from build123d import *

# Parameters (mm, degrees)
SKETCH1_R           = 3.175
BOSS_EXTRUDE1_DEPTH = 66.04
BOSS_EXTRUDE2_START = -2.54
BOSS_EXTRUDE2_DEPTH = 2.54
SKETCH3_R           = 6.35
SKETCH3_R_2         = 3.175
BOSS_EXTRUDE3_DEPTH = 6.35


with BuildPart() as part:
    # Sketch1 → Boss-Extrude1 (new body)
    with BuildSketch(Plane(origin=(0, 0, 0), x_dir=(1, 0, 0), z_dir=(0, 1, 0))):
        with Locations(Location((0, 0, 0), (0, 0, 270))):
            Circle(SKETCH1_R)
    extrude(amount=BOSS_EXTRUDE1_DEPTH)

    # Sketch2 → Boss-Extrude2 (add)
    with BuildSketch(Plane(origin=(0, 66.04, 0), x_dir=(1, 0, 0), z_dir=(0, 1, 0)).offset(BOSS_EXTRUDE2_START)):
        with BuildLine():
            Line((1.27, 4.259709497), (1.27, 2.909935566))
            ThreePointArc((1.27, 2.909935566), (0, 3.175), (-1.27, 2.909935566))
            Line((-1.27, 2.909935566), (-1.27, 4.259709497))
            ThreePointArc((-1.27, 4.259709497), (0, 4.445), (1.27, 4.259709497))
        make_face()
    extrude(amount=BOSS_EXTRUDE2_DEPTH)

    # Sketch3 → Boss-Extrude3 (add)
    with BuildSketch(Plane.XZ):
        with Locations(Location((0, 0, 0), (0, 0, 270))):
            Circle(SKETCH3_R)
        with Locations(Location((0, 0, 0), (0, 0, 270))):
            Circle(SKETCH3_R_2, mode=Mode.SUBTRACT)
    extrude(amount=-BOSS_EXTRUDE3_DEPTH)


solid = part.part
Part model, mm, in its own coordinate system. A direction names the side the tool comes from. Give positions to 0.01 mm unless a question says otherwise; leave off trailing zeros. Order: outer loops, then holes, each group sorted by start corner. A loop starts at its lowest first (then second) coordinate and runs counter-clockwise, first axis right, second up. Notation, with made-up numbers: (-21, -0.5) -> (21, -0.5) arc R13 cw to (21, 24.5) -> close; hole circle Ø3 at (34, 50). An arc over 180 degrees is marked (long way). Use one line per item in the form item = value.
(1) Saw through at A-A (x = 0). Write the cut outline in (y, z) (3 decimals).
Solution:
outline = (0, -6.35) -> (6.35, -6.35) -> (6.35, -3.175) -> (63.5, -3.175) -> (63.5, -4.445) -> (66.04, -4.445) -> (66.04, 3.175) -> (6.35, 3.175) -> (6.35, 6.35) -> (0, 6.35) -> close
(2) Saw through at C-C (y = 16.5). Write the cut outline in (x, z) (3 decimals).
Solution:
outline = circle Ø6.35 at (0, 0)
(3) Tool access for faces 4 (the face through (1.27, 65, -4)), 5 (the face through (0, 0, 0)), 6 (the face through (-1.27, 65, -4)): list every direction of +Z, -Z, +X, -X, +Y, -Y with a clear straight run to the whole face (end or side of a thin tool).
Solution:
face_4 = -Z, +X, +Y
face_5 = +Z, -Z, +X, -X, -Y
face_6 = -Z, -X, +Y
(4) Pull direction Y, two halves, no side cores. Call faces 1 (the face through (-0.018, 64.752, -4.445)), 2 (the face through (0, 66.04, -1)), 3 (the face through (0, 63.5, -4)): +Y half, -Y half, draft (parallel to the pull), parting line (faces both ways), or undercut.
Solution:
face_1 = draft
face_2 = +Y half
face_3 = undercut
(5) Flat gauge pins, fed straight in: P1, Ø4, axis at y = 10, z = -4.5, coming from the +X side; P2, Ø1.5, axis at x = 2.5, y = 15, coming from the +Z side; P3, Ø1, axis at x = 1, y = 35.5, coming from the -Z side. Where does each tip first touch, or does it go through?
Solution:
P1 = 1.96
P2 = 2.65
P3 = -3.14
(6) Drill centre lines: line 1 (Y direction, x = -0.5, z = 4.25); line 2 (X direction, y = 25, z = -0.25); line 3 (X direction, y = 34, z = 0.75). Where is each one in solid material? Low to high. Write a range as from..to.
Solution:
line_1 = 0..6.35
line_2 = -3.17..3.17
line_3 = -3.09..3.09
(7) Saw through at B-B (z = 0). Write the cut outline in (x, y) (3 decimals).
Solution:
outline = (-6.35, 0) -> (6.35, 0) -> (6.35, 6.35) -> (3.175, 6.35) -> (3.175, 66.04) -> (-3.175, 66.04) -> (-3.175, 6.35) -> (-6.35, 6.35) -> close
(8) Saw through at D-D (x = 4.25). Write the cut outline in (y, z).
Solution:
outline = (0, -4.72) -> (6.35, -4.72) -> (6.35, 4.72) -> (0, 4.72) -> close
